The model under review builds one solid part; all positions refer to its coordinate system, in mm. Face numbers are marked on the shaded views. A direction names the side the tool comes from. Round coordinates to 2 decimals unless told otherwise and drop trailing zeros. Write each loop counter-clockwise with the first axis right and the second up, starting at its lowest first coordinate (ties: lowest second). Pieces come first, ordered by that corner, then holes.
Item 1: Clearance check with flat-ended pins moving along their axes: pin 1 Ø10 at (x, y) = (-39, 4.5) entering from -Z; pin 2 Ø14.5 at (x, y) = (-50.546, 9.525) entering from -Z; pin 3 Ø12 at (x, y) = (-53, 11.5) entering from -Z. State where each tip first meets the part, or that it passes through.
Item 2: Machinability: for the marked faces 1, 2, 3 and 4, which of the approach directions +Z, -Z, +X, -X, +Y, -Y give a long, thin tool a straight path to every point of the face, cutting with its end or side? Answer none if there is none.
Item 3: Add section C-C (z = 0). Give the boundary of the cut face in (x, y) (3 decimals), plus the area to 3 significant figures.
Item 4: To check wall thickness, follow L1, parallel to X at y = 27, z = 56; L2, parallel to X at y = 18, z = 59.5; L3, parallel to X at y = 27, z = -34. State the ranges of each line that lie inside material, in increasing order.
Item 5: Draft analysis for pull direction Y (two halves, no side actions). For the marked faces 5, 6 and 7, state which applies: +Y half, -Y half, draft (parallel to the pull), parting line (faces both ways), or undercut.
Item 6: Add section A-A (y = 27). State how many separate pieces and enclosed holes the cut face has, plus the area to 3 significant figures.
Item 7: Add section D-D (z = -39). Give the boundary of the cut face in (x, y).
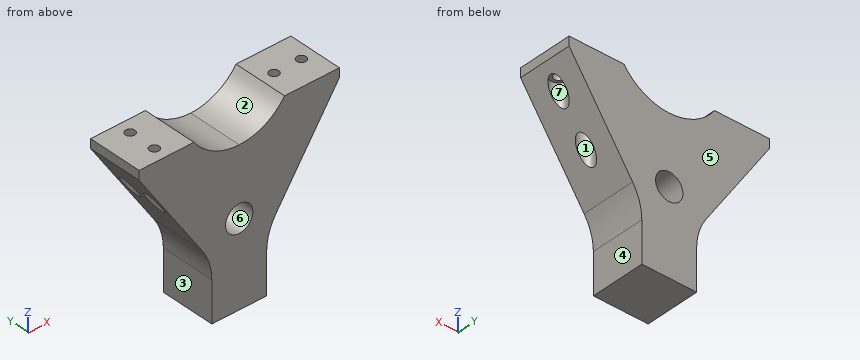
Autodesk Inventor part; units mm, degrees
ref_plane "YZ Plane" through (0, 0, 0) normal (1, 0, 0) x (0, 1, 0)
ref_plane "XZ Plane" through (0, 0, 0) normal (0, 1, 0) x (-1, 0, 0)
ref_plane "XY Plane" through (0, 0, 0) normal (0, 0, 1) x (1, 0, 0)
sketch "Sketch1" plane through (0, 0, 0) normal (0, 1, 0) x (-1, 0, 0)
  line L0 (19.05, -18.5452) -> (19.05, -58.42)
  line L1 (19.05, -58.42) -> (0, -58.42)
  line L2 (19.05, -58.42) -> (19.05, -18.5452)
  line L3 (31.496, 63.5) -> (69.596, 63.5)
  arc A0 (0, 47.0625) -> (31.496, 63.5) centre (0, 85.4562) ccw
  line L4 (0, 85.4562) -> (0, -58.42) construction
  line L5 (69.596, 63.5) -> (69.596, 57.15)
  line L6 (69.596, 57.15) -> (19.05, -18.5452)
  line L7 (0, 0) -> (69.596, 0) construction
  line L8 (-19.05, -58.42) -> (0, -58.42)
  line L9 (-19.05, -58.42) -> (-19.05, -18.5452)
  line L10 (-31.496, 63.5) -> (-69.596, 63.5)
  arc A1 (-31.496, 63.5) -> (0, 47.0625) centre (0, 85.4562) ccw
  line L11 (-69.596, 63.5) -> (-69.596, 57.15)
  line L12 (-69.596, 57.15) -> (-19.05, -18.5452)
  dimension "d73" = 38.3937
  dimension "d74" = 57.15
  dimension "d75" = 18.5452
  dimension "d76" = 19.05
  dimension "d77" = 58.42
  dimension "d78" = 69.596
  dimension "d79" = 38.1
  dimension "d80" = 31.496
  dimension "d81" = 63.5
  dimension "d82" = 6.35
  dimension "d83" = 39.8748
  dimension "d84" = 47.0626
  dimension "d86" = 121.92
  dimension "d90" = 38.1
extrude "Extrusion1" add sketch "Sketch1" along normal blind 38.1
hole "Hole1" at (0, 0, 0) direction (0, 1, 0) diameter 19.05 end through all
sketch "Sketch2" plane through (19.05, 0, -58.42) normal (0, 0, -1) x (-1, 0, 0)
  line L0 (38.1, 0) -> (88.646, 0)
  line L1 (88.646, 0) -> (88.646, 38.1)
  line L2 (38.1, 38.1) -> (88.646, 38.1)
  line L3 (38.1, 0) -> (38.1, 38.1)
  line L4 (-50.546, 0) -> (0, 0)
  line L5 (0, 0) -> (0, 38.1)
  line L6 (-50.546, 38.1) -> (0, 38.1)
  line L7 (-50.546, 0) -> (-50.546, 38.1)
  line L8 (88.646, 0) -> (50.546, 0)
  line L9 (50.546, 0) -> (50.546, 38.1)
  line L10 (88.646, 38.1) -> (50.546, 38.1)
  line L11 (88.646, 0) -> (88.646, 38.1)
  line L12 (69.596, 38.1) -> (69.596, 0) construction
  line L13 (-12.446, 0) -> (-12.446, 38.1) construction
  line L14 (-50.546, 19.05) -> (-12.446, 19.05) construction
  point P0 (19.05, 0)
  point P1 (-41.021, 19.05)
  point P2 (-21.971, 19.05)
  point P3 (69.596, 28.575)
  point P4 (69.596, 9.525)
  dimension "d92" = 38.1
  dimension "d93" = 9.525
  dimension "d94" = 9.525
  dimension "d95" = 9.525
  dimension "d96" = 9.525
  dimension "d97" = 38.1
hole "Hole2" at (60.071, 19.05, -58.42) at (41.021, 19.05, -58.42) at (-50.546, 28.575, -58.42) at (-50.546, 9.525, -58.42) direction (0, 0, 1) diameter 6.5278 depth 121.92 counterbore diameter 11.1252 counterbore depth 110.49
fillet "Fillet1" radius 38.1 2 edges at (19.05, 19.05, -18.5452) (-19.05, 19.05, -18.5452)
properties part number "front leg"
Numbers:
1. pin 1: stops at z = 3.84
1. pin 2: stops at z = 17.76
1. pin 3: stops at z = 24.35
2. face 1: -Z
2. face 2: +Z, +Y, -Y
2. face 3: -Z, -X, +Y, -Y
2. face 4: -Z, +X, +Y, -Y
3. outline: (-31.434, 0) - (-9.525, 0) - (-9.525, 38.1) - (-31.434, 38.1) - close; (9.525, 0) - (31.434, 0) - (31.434, 38.1) - (9.525, 38.1) - close
3. area: 1,670 mm2
4. L1: x = -68.83 to -53.4, -47.69 to -24.63, 24.63 to 68.83
4. L2: x = -69.6 to -28.29, 28.29 to 37.93, 44.11 to 56.98, 63.16 to 69.6
4. L3: x = -19.05 to 19.05
5. face 5: +Y half
5. face 6: draft
5. face 7: undercut
6. separate pieces: 2
6. enclosed holes: 1
6. area: 7,810 mm2
7. outline: (-19.05, 0) - (19.05, 0) - (19.05, 38.1) - (-19.05, 38.1) - close
